from build123d import *

# Parameters (mm, degrees)
F0_W     = 52.483174
F0_H     = 39.362366
F1_DEPTH = 12.7
F3_DEPTH = 52.484174
F4_R     = 17.52473
F4_R_2   = 14.98473
F5_DEPTH = 12.7
F6_DEPTH = 19.05
F7_DEPTH = 25.4


with BuildPart() as f1:
    # F0 (on Front) → F1 (new body)
    with BuildSketch(Plane.XZ):
        Rectangle(F0_W, F0_H)
    extrude(amount=F1_DEPTH)

    # F2 (on face) → F3 (cut, through all)
    with BuildSketch(Plane(origin=(-26.241587, 0, 0), x_dir=(0, -1, 0), z_dir=(-1, 0, 0))):
        Polygon((6.35, 19.681183), (3.175, 19.681183), (3.175, -19.681183), (6.35, -19.681183), (9.525, -19.681183), (9.525, 19.681183), align=None)
    extrude(amount=-F3_DEPTH, mode=Mode.SUBTRACT)

    # F4 (on face) → F5 (join)
    with BuildSketch(Plane.XZ.offset(12.7)):
        with BuildLine():
            ThreePointArc((-19.196799, 15.615331), (-19.75476, 16.962369), (-21.101799, 17.520331))
            Line((-21.101799, 17.520331), (-21.101799, 15.615331))
            Line((-21.101799, 15.615331), (-21.101799, 13.710331))
            ThreePointArc((-21.101799, 13.710331), (-19.75476, 14.268293), (-19.196799, 15.615331))
        make_face()
        with BuildLine():
            ThreePointArc((-19.196799, -15.615332), (-19.75476, -14.268294), (-21.101799, -13.710332))
            Line((-21.101799, -13.710332), (-21.101799, -15.615332))
            Line((-21.101799, -15.615332), (-21.101799, -17.520332))
            ThreePointArc((-21.101799, -17.520332), (-19.75476, -16.96237), (-19.196799, -15.615332))
        make_face()
        with BuildLine():
            Line((-21.101799, -15.615332), (-21.101799, -13.710332))
            ThreePointArc((-21.101799, -13.710332), (-23.006799, -15.615332), (-21.101799, -17.520332))
            Line((-21.101799, -17.520332), (-21.101799, -15.615332))
        make_face()
        with BuildLine():
            Line((-21.101799, 15.615331), (-21.101799, 17.520331))
            ThreePointArc((-21.101799, 17.520331), (-23.006799, 15.615331), (-21.101799, 13.710331))
            Line((-21.101799, 13.710331), (-21.101799, 15.615331))
        make_face()
        with BuildLine():
            ThreePointArc((23.006799, 15.615331), (22.448837, 16.962369), (21.101799, 17.520331))
            Line((21.101799, 17.520331), (21.101799, 15.615331))
            Line((21.101799, 15.615331), (21.101799, 13.710331))
            ThreePointArc((21.101799, 13.710331), (22.448837, 14.268293), (23.006799, 15.615331))
        make_face()
        with BuildLine():
            ThreePointArc((23.006799, -15.615332), (22.448837, -14.268294), (21.101799, -13.710332))
            Line((21.101799, -13.710332), (21.101799, -15.615332))
            Line((21.101799, -15.615332), (21.101799, -17.520332))
            ThreePointArc((21.101799, -17.520332), (22.448837, -16.96237), (23.006799, -15.615332))
        make_face()
        with BuildLine():
            Line((21.101799, -15.615332), (21.101799, -13.710332))
            ThreePointArc((21.101799, -13.710332), (19.196799, -15.615332), (21.101799, -17.520332))
            Line((21.101799, -17.520332), (21.101799, -15.615332))
        make_face()
        with BuildLine():
            Line((21.101799, 15.615331), (21.101799, 17.520331))
            ThreePointArc((21.101799, 17.520331), (19.196799, 15.615331), (21.101799, 13.710331))
            Line((21.101799, 13.710331), (21.101799, 15.615331))
        make_face()
        with Locations((0, 1.094137)):
            Circle(F4_R)
        with Locations((0, 1.094137)):
            Circle(F4_R_2, mode=Mode.SUBTRACT)
    extrude(amount=-F5_DEPTH)

    # F4 (on face) → F6 (join)
    with BuildSketch(Plane.XZ.offset(12.7)):
        with Locations((0, 1.094137)):
            Circle(F4_R)
        with Locations((0, 1.094137)):
            Circle(F4_R_2, mode=Mode.SUBTRACT)
    extrude(amount=F6_DEPTH)

    # F4 (on face) → F7 (cut)
    with BuildSketch(Plane.XZ.offset(12.7)):
        with Locations((0, 1.094137)):
            Circle(F4_R_2)
    extrude(amount=-F7_DEPTH, mode=Mode.SUBTRACT)


solid = f1.part
Work out the finished part from the listing and answer in its coordinate system (mm). A direction names the side the tool comes from. Give positions to 0.01 mm unless a question says otherwise; leave off trailing zeros. Write each loop counter-clockwise with the first axis right and the second up, starting at its lowest first coordinate (ties: lowest second). Pieces come first, ordered by that corner, then holes. Notation, with made-up numbers: (70.5, 55.25) - (77.5, 55.25) arc R25 cw to (77.5, 76.25) - close; hole circle Ø3 at (-25.5, 60.25). An arc over 180 degrees is marked (long way). One line per item, written item: value. Start each with the question number.
1. Find section B-B (y = -7). Write down the section's boundary in (x, z) (3 decimals).
2. Find section A-A (x = 0). Write down the section's boundary in (y, z) (3 decimals), then the cut area to 3 significant figures.
3. Given pin 1 (6 mm diameter, centred on y = -18.5, z = 9.5, fed in from +X); pin 2 (4 mm diameter, centred on y = -25.5, z = 4.5, fed in from -X); pin 3 (10 mm diameter, centred on x = 7, z = -2.5, fed in from +Y); pin 4 (6 mm diameter, centred on x = -6, y = -22.5, fed in from -Z), each flat-ended and moving along its own axis, determine where each tip first touches the part or whether it passes through.
4. For faces 5 (the flat face through (0, -9.525, -18)), 6 (the flat face through (0, -2, 19.681)), determine the directions among +Z, -Z, +X, -X, +Y, -Y from which every point of the face is accessible in a straight line to the end or side of a thin tool.
5. Find section D-D (y = -27.5). Write down the section's boundary in (x, z).
6. For a pull along X with two mould halves and no side action, classify faces 1 (the flat face through (-12, -12.7, -13)), 2 (the cylindrical face through (16.715, -22.092, 6.358)), 3 (the flat face through (-26.242, -2, 0)), 4 (the cylindrical face through (16.715, -6.394, 6.358)) as +X half, -X half, draft (parallel to the pull), parting line (faces both ways), or undercut.
7. Find section C-C (z = 8). Write down the section's boundary in (x, y) (3 decimals).
8. Consider probe 1 along Y at (x, z) = (9, -15) (3 decimals); probe 2 along Z at (x, y) = (0, -2); probe 3 along Z at (x, y) = (0, -22). Determine where each line is inside the solid, lowest interval first.
Geometry results:
1. outline: circle Ø3.81 at (-21.102, -15.615); circle Ø3.81 at (-21.102, 15.615); circle Ø35.049 at (0, 1.094); (21.102, -17.52) arc R1.905 ccw to (23.007, -15.615) arc R1.905 ccw to (21.102, -13.71) arc R1.905 ccw to start; (21.102, 13.71) arc R1.905 ccw to (23.007, 15.615) arc R1.905 ccw to (21.102, 17.52) arc R1.905 ccw to start; hole circle Ø29.969 at (0, 1.094)
2. outline: (-31.75, -16.431) - (-12.7, -16.431) - (-12.7, -19.681) - (-9.525, -19.681) - (-9.525, -16.431) - (-3.175, -16.431) - (-3.175, -19.681) - (0, -19.681) - (0, -13.891) - (-31.75, -13.891) - close; (-31.75, 16.079) - (0, 16.079) - (0, 19.681) - (-3.175, 19.681) - (-3.175, 18.619) - (-9.525, 18.619) - (-9.525, 19.681) - (-12.7, 19.681) - (-12.7, 18.619) - (-31.75, 18.619) - close
2. area: 189 mm2
3. pin 1: x = 16.67
3. pin 2: x = -17.47
3. pin 3: through
3. pin 4: z = -16.17
4. face 5: none
4. face 6: +Z, +X, -X, +Y, -Y
5. outline: circle Ø35.05 at (0, 1.09); hole circle Ø29.97 at (0, 1.09)
6. face 1: draft
6. face 2: parting line
6. face 3: -X half
6. face 4: undercut
7. outline: (-26.242, -12.7) - (-16.107, -12.7) - (-16.107, -31.75) - (-13.299, -31.75) - (-13.299, 0) - (-26.242, 0) - (-26.242, -3.175) - (-16.107, -3.175) - (-16.107, -9.525) - (-26.242, -9.525) - close; (13.299, -31.75) - (16.107, -31.75) - (16.107, -12.7) - (26.242, -12.7) - (26.242, -9.525) - (16.107, -9.525) - (16.107, -3.175) - (26.242, -3.175) - (26.242, 0) - (13.299, 0) - close
8. probe 1: -12.7 to -9.525, -3.175 to 0
8. probe 2: -19.68 to -13.89, 16.08 to 19.68
8. probe 3: -16.43 to -13.89, 16.08 to 18.62
